Here's how the part is built. I have some questions about the finished solid (model axes, mm). Face numbers are marked on the shaded views. A direction names the side the tool comes from. Coordinates: 2 decimals unless noted, no trailing zeros. Order: outer loops, then holes, each group sorted by start corner. A loop starts at its lowest first (then second) coordinate and runs counter-clockwise, first axis right, second up. Notation, with made-up numbers: (44.25, 19.25) - (67.25, 19.25) arc R23 ccw to (67.25, 31.25) - close; hole circle Ø2 at (12, 70). An arc over 180 degrees is marked (long way). Use CSV: the item, a comma, the result in double quotes. Start each with the question number.
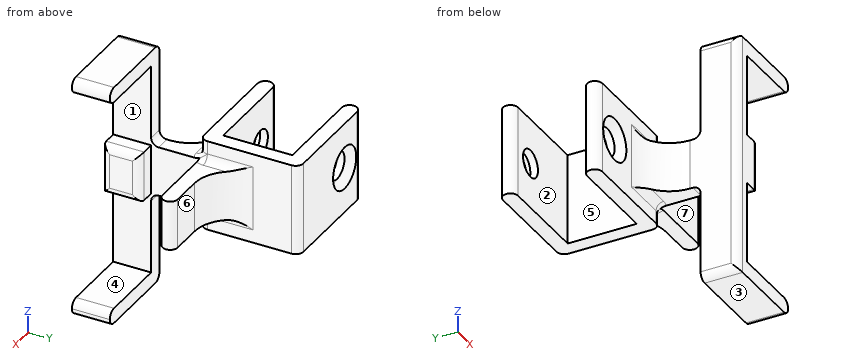
from build123d import *

# Parameters (mm, degrees)
SKETCH1_W               = 10
SKETCH1_H               = 2
BOSS_EXTRUDE1_DEPTH     = 3.275
BOSS_EXTRUDE2_DEPTH     = 6
SKETCH3_W               = 2
SKETCH3_H               = 5
BOSS_EXTRUDE3_DEPTH     = 16
SKETCH4_W               = 2
SKETCH4_H               = 5
BOSS_EXTRUDE4_DEPTH     = 10
FILLET1_R               = 1
FILLET2_R               = 1
CUT_EXTRUDE1_DEPTH      = 33.01952537
CUT_EXTRUDE1_DEPTH_BACK = 33.01952537
SKETCH2_R               = 1.8
CHAMFER1_SIZE           = 1
FILLET3_R               = 5


with BuildPart() as part:
    # Sketch1 → Boss-Extrude1 (new, symmetric)
    with BuildSketch(Plane.XY):
        Polygon((0, -9.1), (-13, -9.1), (-13, -11.1), (2, -11.1), (2, 2), (-13, 2), (-13, 0), (0, 0), align=None)
        Polygon((2, -11.1), (0, -11.1), (0, -22.5), (4.7, -22.5), (4.7, -17.5), (2, -17.5), align=None)
        with Locations((7, -10.1)):
            Rectangle(SKETCH1_W, SKETCH1_H)
    extrude(amount=BOSS_EXTRUDE1_DEPTH, both=True)

    # Sketch1<3> → Boss-Extrude2 (add, symmetric)
    with BuildSketch(Plane.XY):
        Polygon((0, -9.1), (-13, -9.1), (-13, -11.1), (2, -11.1), (2, 2), (-13, 2), (-13, 0), (0, 0), align=None)
    extrude(amount=BOSS_EXTRUDE2_DEPTH, both=True)

    # Sketch3 → Boss-Extrude3 (add, symmetric)
    with BuildSketch(Plane.XY):
        with Locations((1, -20)):
            Rectangle(SKETCH3_W, SKETCH3_H)
    extrude(amount=BOSS_EXTRUDE3_DEPTH, both=True)

    # Sketch4 → Boss-Extrude4 (add)
    with BuildSketch(Plane(origin=(2, 0, 0), x_dir=(0, 0, -1), z_dir=(1, 0, 0))):
        with Locations((-15, -20)):
            Rectangle(SKETCH4_W, SKETCH4_H)
        with Locations((15, -20)):
            Rectangle(SKETCH4_W, SKETCH4_H)
    extrude(amount=BOSS_EXTRUDE4_DEPTH)

    # Fillet1
    # the kernel refuses this fillet: 1 mm, written as the material it adds along each edge
    with BuildSketch(Plane(origin=(2, -17.5, 3.275), x_dir=(0, 1, 0), z_dir=(-1, 0, 0)), Plane(origin=(2, -17.5, -3.275), x_dir=(0, 0, -1), z_dir=(-1, 0, 0))) as fillet1_piece_1:
        with BuildLine():
            CenterArc((FILLET1_R, -FILLET1_R), FILLET1_R, 90, 90)
            Line((0, -FILLET1_R), (0, 0))
            Line((0, 0), (FILLET1_R, 0))
        make_face()
    extrude(amount=2)
    # the kernel refuses this fillet: 1 mm, written as the material it takes off along each edge
    with BuildSketch(Plane(origin=(-13, -9.1, -8.5), x_dir=(1, 0, 0), z_dir=(0, 0, 1)), Plane(origin=(-13, -11.1, -8.5), x_dir=(0, 1, 0), z_dir=(0, 0, 1)), Plane(origin=(2, 2, -8.5), x_dir=(0, -1, 0), z_dir=(0, 0, 1)), Plane(origin=(-13, 2, -8.5), x_dir=(1, 0, 0), z_dir=(0, 0, 1))) as fillet1_2_piece_1:
        with BuildLine():
            CenterArc((FILLET1_R, -FILLET1_R), FILLET1_R, 90, 90)
            Line((0, -FILLET1_R), (0, 0))
            Line((0, 0), (FILLET1_R, 0))
        make_face()
    extrude(amount=17, mode=Mode.SUBTRACT)
    with BuildSketch(Plane(origin=(2, -11.1, -8.5), x_dir=(-1, 0, 0), z_dir=(0, 0, 1)), Plane(origin=(2, -11.1, 3.275), x_dir=(-1, 0, 0), z_dir=(0, 0, 1))) as fillet1_2_piece_2:
        with BuildLine():
            CenterArc((FILLET1_R, -FILLET1_R), FILLET1_R, 90, 90)
            Line((0, -FILLET1_R), (0, 0))
            Line((0, 0), (FILLET1_R, 0))
        make_face()
    extrude(amount=5.225, mode=Mode.SUBTRACT)
    with BuildSketch(Plane(origin=(12, -15, 14), x_dir=(-1, 0, 0), z_dir=(0, -1, 0)), Plane(origin=(12, -15, -14), x_dir=(0, 0, -1), z_dir=(0, -1, 0)), Plane(origin=(0, -15, -16), x_dir=(0, 0, 1), z_dir=(0, -1, 0)), Plane(origin=(12, -25, 16), x_dir=(-1, 0, 0), z_dir=(0, 1, 0))) as fillet1_2_piece_3:
        with BuildLine():
            CenterArc((FILLET1_R, -FILLET1_R), FILLET1_R, 90, 90)
            Line((0, -FILLET1_R), (0, 0))
            Line((0, 0), (FILLET1_R, 0))
        make_face()
    extrude(amount=10, mode=Mode.SUBTRACT)
    with BuildSketch(Plane(origin=(0, -22.5, -18.5), x_dir=(0, 1, 0), z_dir=(0, 0, 1))) as fillet1_2_piece_4:
        with BuildLine():
            CenterArc((FILLET1_R, -FILLET1_R), FILLET1_R, 90, 90)
            Line((0, -FILLET1_R), (0, 0))
            Line((0, 0), (FILLET1_R, 0))
        make_face()
    extrude(amount=37, mode=Mode.SUBTRACT)
    with BuildSketch(Plane(origin=(4.7, -22.5, -5.775), x_dir=(-1, 0, 0), z_dir=(0, 0, 1)), Plane(origin=(4.7, -17.5, 5.775), x_dir=(-1, 0, 0), z_dir=(0, 0, -1))) as fillet1_2_piece_5:
        with BuildLine():
            CenterArc((FILLET1_R, -FILLET1_R), FILLET1_R, 90, 90)
            Line((0, -FILLET1_R), (0, 0))
            Line((0, 0), (FILLET1_R, 0))
        make_face()
    extrude(amount=11.55, mode=Mode.SUBTRACT)
    with BuildSketch(Plane(origin=(4.7, -25, 3.275), x_dir=(0, 0, -1), z_dir=(0, 1, 0)), Plane(origin=(4.7, -25, -3.275), x_dir=(-1, 0, 0), z_dir=(0, 1, 0)), Plane(origin=(12, -25, -16), x_dir=(-1, 0, 0), z_dir=(0, 1, 0)), Plane(origin=(0, -15, 16), x_dir=(0, 0, -1), z_dir=(0, -1, 0))) as fillet1_2_piece_6:
        with BuildLine():
            CenterArc((FILLET1_R, FILLET1_R), FILLET1_R, 180, 90)
            Line((0, FILLET1_R), (0, 0))
            Line((0, 0), (FILLET1_R, 0))
        make_face()
    extrude(amount=10, mode=Mode.SUBTRACT)
    with BuildSketch(Plane(origin=(12, -11.1, -5.775), x_dir=(0, 1, 0), z_dir=(0, 0, 1)), Plane(origin=(12, -9.1, -5.775), x_dir=(-1, 0, 0), z_dir=(0, 0, 1))) as fillet1_2_piece_7:
        with BuildLine():
            CenterArc((FILLET1_R, FILLET1_R), FILLET1_R, 180, 90)
            Line((0, FILLET1_R), (0, 0))
            Line((0, 0), (FILLET1_R, 0))
        make_face()
    extrude(amount=11.55, mode=Mode.SUBTRACT)
    with BuildSketch(Plane(origin=(-13, 0, 8.5), x_dir=(0, 1, 0), z_dir=(0, 0, -1))) as fillet1_2_piece_8:
        with BuildLine():
            CenterArc((FILLET1_R, FILLET1_R), FILLET1_R, 180, 90)
            Line((0, FILLET1_R), (0, 0))
            Line((0, 0), (FILLET1_R, 0))
        make_face()
    extrude(amount=17, mode=Mode.SUBTRACT)

    # Fillet2
    # the kernel refuses this fillet: 1 mm, written as the material it adds along each edge
    with BuildSketch(Plane(origin=(1, -10.1, -3.275), x_dir=(0, -1, 0), z_dir=(-1, 0, 0))) as fillet2_piece_1_section:
        with BuildLine():
            CenterArc((1 + FILLET2_R, -FILLET2_R), FILLET2_R, 90, 90)
            Line((1, -FILLET2_R), (1, 0))
            Line((1, 0), (1 + FILLET2_R, 0))
        make_face()
    fillet2_piece_1 = revolve(axis=Axis((1, -10.1, -3.275), (0, 0, 1)), revolution_arc=90, mode=Mode.PRIVATE)
    fillet2_piece_1 = split(fillet2_piece_1, bisect_by=Plane(origin=(2, -11.34730941, -3.421981112), z_dir=(-1, 0, 0)), keep=Keep.TOP, mode=Mode.PRIVATE)
    fillet2_piece_1 = split(fillet2_piece_1, bisect_by=Plane(origin=(1.400007142, -11.1, -3.421981112), z_dir=(0, -1, 0)), keep=Keep.TOP, mode=Mode.PRIVATE)
    add(fillet2_piece_1)
    with BuildSketch(Plane(origin=(1, -10.1, -3.275), x_dir=(0, -1, 0), z_dir=(-1, 0, 0))) as fillet2_piece_2_section:
        with BuildLine():
            CenterArc((1 + FILLET2_R, -FILLET2_R), FILLET2_R, 90, 90)
            Line((1, -FILLET2_R), (1, 0))
            Line((1, 0), (1 + FILLET2_R, 0))
        make_face()
    fillet2_piece_2 = revolve(axis=Axis((1, -10.1, -3.275), (0, 0, 1)), revolution_arc=90, mode=Mode.PRIVATE)
    fillet2_piece_2 = split(fillet2_piece_2, bisect_by=Plane(origin=(2, -10.826426326, -3.613950845), z_dir=(-1, 0, 0)), keep=Keep.TOP, mode=Mode.PRIVATE)
    fillet2_piece_2 = split(fillet2_piece_2, bisect_by=Plane(origin=(1.726426326, -11.1, -3.613950845), z_dir=(0, 1, 0)), keep=Keep.TOP, mode=Mode.PRIVATE)
    add(fillet2_piece_2)
    with BuildSketch(Plane(origin=(1, -10.1, -3.275), x_dir=(0, -1, 0), z_dir=(-1, 0, 0))) as fillet2_piece_3_section:
        with BuildLine():
            CenterArc((1 + FILLET2_R, -FILLET2_R), FILLET2_R, 90, 90)
            Line((1, -FILLET2_R), (1, 0))
            Line((1, 0), (1 + FILLET2_R, 0))
        make_face()
    fillet2_piece_3 = revolve(axis=Axis((1, -10.1, -3.275), (0, 0, 1)), revolution_arc=90, mode=Mode.PRIVATE)
    fillet2_piece_3 = split(fillet2_piece_3, bisect_by=Plane(origin=(2, -10.500007075, -3.421981186), z_dir=(1, 0, 0)), keep=Keep.TOP, mode=Mode.PRIVATE)
    fillet2_piece_3 = split(fillet2_piece_3, bisect_by=Plane(origin=(2.24730905, -11.1, -3.421981186), z_dir=(0, 1, 0)), keep=Keep.TOP, mode=Mode.PRIVATE)
    add(fillet2_piece_3)
    with BuildSketch(Plane(origin=(1, -10.1, 3.275), x_dir=(0, -1, 0), z_dir=(-1, 0, 0))) as fillet2_piece_4_section:
        with BuildLine():
            CenterArc((1 + FILLET2_R, FILLET2_R), FILLET2_R, 180, 90)
            Line((1, FILLET2_R), (1, 0))
            Line((1, 0), (1 + FILLET2_R, 0))
        make_face()
    fillet2_piece_4 = revolve(axis=Axis((1, -10.1, 3.275), (0, 0, 1)), revolution_arc=90, mode=Mode.PRIVATE)
    fillet2_piece_4 = split(fillet2_piece_4, bisect_by=Plane(origin=(2, -11.34730941, 3.421981112), z_dir=(-1, 0, 0)), keep=Keep.TOP, mode=Mode.PRIVATE)
    fillet2_piece_4 = split(fillet2_piece_4, bisect_by=Plane(origin=(1.400007142, -11.1, 3.421981112), z_dir=(0, -1, 0)), keep=Keep.TOP, mode=Mode.PRIVATE)
    add(fillet2_piece_4)
    with BuildSketch(Plane(origin=(1, -10.1, 3.275), x_dir=(0, -1, 0), z_dir=(-1, 0, 0))) as fillet2_piece_5_section:
        with BuildLine():
            CenterArc((1 + FILLET2_R, FILLET2_R), FILLET2_R, 180, 90)
            Line((1, FILLET2_R), (1, 0))
            Line((1, 0), (1 + FILLET2_R, 0))
        make_face()
    fillet2_piece_5 = revolve(axis=Axis((1, -10.1, 3.275), (0, 0, 1)), revolution_arc=90, mode=Mode.PRIVATE)
    fillet2_piece_5 = split(fillet2_piece_5, bisect_by=Plane(origin=(2, -10.826426326, 3.613950845), z_dir=(-1, 0, 0)), keep=Keep.TOP, mode=Mode.PRIVATE)
    fillet2_piece_5 = split(fillet2_piece_5, bisect_by=Plane(origin=(1.726426326, -11.1, 3.613950845), z_dir=(0, 1, 0)), keep=Keep.TOP, mode=Mode.PRIVATE)
    add(fillet2_piece_5)
    with BuildSketch(Plane(origin=(1, -10.1, 3.275), x_dir=(0, -1, 0), z_dir=(-1, 0, 0))) as fillet2_piece_6_section:
        with BuildLine():
            CenterArc((1 + FILLET2_R, FILLET2_R), FILLET2_R, 180, 90)
            Line((1, FILLET2_R), (1, 0))
            Line((1, 0), (1 + FILLET2_R, 0))
        make_face()
    fillet2_piece_6 = revolve(axis=Axis((1, -10.1, 3.275), (0, 0, 1)), revolution_arc=90, mode=Mode.PRIVATE)
    fillet2_piece_6 = split(fillet2_piece_6, bisect_by=Plane(origin=(2, -10.500007075, 3.421981186), z_dir=(1, 0, 0)), keep=Keep.TOP, mode=Mode.PRIVATE)
    fillet2_piece_6 = split(fillet2_piece_6, bisect_by=Plane(origin=(2.24730905, -11.1, 3.421981186), z_dir=(0, 1, 0)), keep=Keep.TOP, mode=Mode.PRIVATE)
    add(fillet2_piece_6)
    with BuildSketch(Plane(origin=(0, -11.1, 3.275), x_dir=(0, -1, 0), z_dir=(1, 0, 0)), Plane(origin=(2, -10.1, 3.275), x_dir=(1, 0, 0), z_dir=(0, 1, 0)), Plane(origin=(0, -11.1, -3.275), x_dir=(0, 0, -1), z_dir=(1, 0, 0)), Plane(origin=(2, -10.1, -3.275), x_dir=(0, 0, -1), z_dir=(0, 1, 0))) as fillet2_piece_7:
        with BuildLine():
            CenterArc((FILLET2_R, -FILLET2_R), FILLET2_R, 90, 90)
            Line((0, -FILLET2_R), (0, 0))
            Line((0, 0), (FILLET2_R, 0))
        make_face()
    extrude(amount=1)

    # Sketch2 → Cut-Extrude1 (cut, two sides: drawn at the far end of the back side and taken through both)
    with BuildSketch(Plane(origin=(0, 2, 0), x_dir=(1, 0, 0), z_dir=(0, 1, 0)).offset(-CUT_EXTRUDE1_DEPTH_BACK)):
        with Locations((-9, 0)):
            Circle(SKETCH2_R)
    extrude(amount=CUT_EXTRUDE1_DEPTH + CUT_EXTRUDE1_DEPTH_BACK, mode=Mode.SUBTRACT)

    # Chamfer1
    chamfer1_edges = [part.edges().sort_by_distance(p)[0] for p in [
        (-10.8, -11.1, 0),
        (-10.8, 2, 0),
    ]]
    chamfer(chamfer1_edges, length=CHAMFER1_SIZE)

    # Fillet3
    fillet3_edges = [part.edges().sort_by_distance(p)[0] for p in [
        (0, -11.1, 0),
        (2, -9.1, 0),
    ]]
    fillet(fillet3_edges, radius=FILLET3_R)


solid = part.part
Item 1: For the marked faces 5, 6 and 7, which set-ups out of +Z, -Z, +X, -X, +Y, -Y let a thin tool reach every point of the face, with its end or its side?
Item 2: Please list where these lines run through material, in increasing order: line 1 along Z through (x, y) = (-9, -9.45); line 2 along Y through (x, z) = (-6, -5.5); line 3 along Z through (x, y) = (4.75, -21.25). Write a range as from..to.
Item 3: For pin 1 Ø3.5 at (x, z) = (8.5, 11) entering from +Y; pin 2 Ø1.2 at (x, y) = (0, -14) entering from +Z (3 decimals); pin 3 Ø4.5 at (x, z) = (8, -1.5) entering from +Y; pin 4 Ø3 at (x, z) = (9, 4) entering from +Y, each with a flat end and sliding along its axis, tell me the tip position at first contact or that it passes through.
Item 4: Suppose I cut it at B-B on x = -5.5. Write out the boundary of the cut face in (y, z), then the cut area to 3 significant figures.
Item 5: We'd pull the mould along Z, two halves only. Please class the marked faces 1, 2, 3 and 4: released by +Z, released by -Z, zero draft, split by the parting line, or undercut.
Item 6: Suppose I cut it at D-D on y = -19. Write out the boundary of the cut face in (x, z) (3 decimals), then the cut area to 3 significant figures.
Item 7: Suppose I cut it at C-C on z = 0. State how many separate pieces and enclosed holes the cut face has, then the cut area to 3 significant figures.
Item 8: Suppose I cut it at A-A on x = 8.75. Write out the boundary of the cut face in (y, z) (3 decimals), then the cut area to 3 significant figures.
Here are the results:
1,face 5,"+Z, -Z, -X"
1,face 6,"+Z, -Z, +X, +Y"
1,face 7,"+Z, -Z, +X"
2,line 1,"-6..-1.8, 1.8..6"
2,line 2,"-11.1..-9.1, 0..2"
2,line 3,"-16..-14, 14..16"
3,pin 1,"through"
3,pin 2,"z = 3.275"
3,pin 3,"y = -8.94"
3,pin 4,"y = -9.1"
4,outline,"(-11.1, -6) - (-9.1, -6) - (-9.1, 6) - (-11.1, 6) - close; (0, -6) - (2, -6) - (2, 6) - (0, 6) - close"
4,area,"48.0 mm^2"
5,face 1,"undercut"
5,face 2,"zero draft"
5,face 3,"released by -Z"
5,face 4,"undercut"
6,outline,"(0, -15) arc R1 ccw to (1, -16) - (11, -16) arc R1 ccw to (11, -14) - (2, -14) - (2, -3.275) - (3.7, -3.275) arc R1 ccw to (4.7, -2.275) - (4.7, 2.275) arc R1 ccw to (3.7, 3.275) - (2, 3.275) - (2, 14) - (11, 14) arc R1 ccw to (11, 16) - (1, 16) arc R1 ccw to (0, 15) - close"
6,area,"120 mm^2"
7,separate pieces,"3"
7,enclosed holes,"0"
7,area,"127 mm^2"
8,outline,"(-22.5, -16) - (-17.5, -16) - (-17.5, -14) - (-22.5, -14) - close; (-22.5, 14) - (-17.5, 14) - (-17.5, 16) - (-22.5, 16) - close; (-11.1, -3.275) - (-9.1, -3.275) - (-9.1, 3.275) - (-11.1, 3.275) - close"
8,area,"33.1 mm^2"
